Build history of the part. All positions in model axes, mm. A direction names the side the tool comes from. Round coordinates to 2 decimals unless told otherwise and drop trailing zeros. Write each loop counter-clockwise with the first axis right and the second up, starting at its lowest first coordinate (ties: lowest second). Pieces come first, ordered by that corner, then holes. Notation, with made-up numbers: (85, 84.5) - (116, 84.5) arc R10 cw to (116, 88.5) - close; hole circle Ø1 at (54, 15.5). An arc over 180 degrees is marked (long way). Answer as a JSON object with one key per item and string values. Group by question number.
Item 1: Slice it at A-A, the plane z = 0. List the corners of the cut face in (x, y) (3 decimals).
Item 2: Slice it at C-C, the plane x = 1.3. List the corners of the cut face in (y, z), then the cut area to 3 significant figures.
Item 3: Slice it at D-D, the plane y = -1.5. List the corners of the cut face in (x, z) (3 decimals), then the cut area to 3 significant figures.
Item 4: Which spindle directions (+Z, -Z, +X, -X, +Y, -Y) get a long thin tool onto all of the face, cutting with end or side? Do faces 4 (the flat face through (0, -2.8, 0)), 5 (the cylindrical face through (-0.75, 5.31, -0.03)), 6 (the cylindrical face through (1.092, -1.38, 0.344)), 7 (the flat face through (0, 7.2, 0)), 8 (the cylindrical face through (-1.4, 3.7, -0.06)). Say none if no direction does.
Item 5: Slice it at B-B, the plane z = 0.95. List the corners of the cut face in (x, y), then the cut area to 3 significant figures.
Item 6: Probe line 1 (Y direction, x = 0.9, z = 0.05); line 2 (Y direction, x = -1.2, z = -0.65); line 3 (Y direction, x = 1.8, z = 0.3). List the from-to ranges inside material, lowest first. Write a range as from..to.
Item 7: Flat gauge pins, fed straight in: pin 1 (1 mm diameter, centred on y = 0, z = 1, fed in from +X); pin 2 (1 mm diameter, centred on x = -1, z = -1.5, fed in from -Y); pin 3 (1.5 mm diameter, centred on y = 3.5, z = -0.5, fed in from -X). Where does each tip first touch, or does it go through?
Item 8: Two-plate mould, pull along Y, no slides. Class faces 1 (the cylindrical face through (-0.434, 0.345, 1.952)), 2 (the flat face through (0, 3.95, 1)), 3 (the flat face through (1, 0, 1)): +Y half, -Y half, draft (parallel to the pull), parting line (faces both ways), or undercut.
from build123d import *

# Parameters (mm, degrees)
SKETCH1_R           = 2
BOSS_EXTRUDE1_DEPTH = 0.7
SKETCH2_R           = 0.75
BOSS_EXTRUDE2_DEPTH = 2.75
SKETCH3_R           = 1.4
BOSS_EXTRUDE3_DEPTH = 0.5
SKETCH4_R           = 0.75
BOSS_EXTRUDE4_DEPTH = 2.75
SKETCH5_R           = 1.4
BOSS_EXTRUDE5_DEPTH = 0.5
SKETCH6_R           = 1.145
BOSS_EXTRUDE6_DEPTH = 2.8


with BuildPart() as part:
    # Sketch1 → Boss-Extrude1 (new body)
    with BuildSketch(Plane(origin=(0, 0, 0), x_dir=(1, 0, 0), z_dir=(0, 1, 0))):
        Circle(SKETCH1_R)
    extrude(amount=BOSS_EXTRUDE1_DEPTH)

    # Sketch2 → Boss-Extrude2 (add)
    with BuildSketch(Plane(origin=(0, 0.7, 0), x_dir=(1, 0, 0), z_dir=(0, 1, 0))):
        Circle(SKETCH2_R)
    extrude(amount=BOSS_EXTRUDE2_DEPTH)

    # Sketch3 → Boss-Extrude3 (add)
    with BuildSketch(Plane(origin=(0, 3.45, 0), x_dir=(1, 0, 0), z_dir=(0, 1, 0))):
        Circle(SKETCH3_R)
    extrude(amount=BOSS_EXTRUDE3_DEPTH)

    # Sketch4 → Boss-Extrude4 (add)
    with BuildSketch(Plane(origin=(0, 3.95, 0), x_dir=(1, 0, 0), z_dir=(0, 1, 0))):
        Circle(SKETCH4_R)
    extrude(amount=BOSS_EXTRUDE4_DEPTH)

    # Sketch5 → Boss-Extrude5 (add)
    with BuildSketch(Plane(origin=(0, 6.7, 0), x_dir=(1, 0, 0), z_dir=(0, 1, 0))):
        Circle(SKETCH5_R)
    extrude(amount=BOSS_EXTRUDE5_DEPTH)

    # Sketch6 → Boss-Extrude6 (add)
    with BuildSketch(Plane.XZ):
        Circle(SKETCH6_R)
    extrude(amount=BOSS_EXTRUDE6_DEPTH)


solid = part.part
Geometry says:
{
 "1": {"outline": "(-2, 0) - (-1.145, 0) - (-1.145, -2.8) - (1.145, -2.8) - (1.145, 0) - (2, 0) - (2, 0.7) - (0.75, 0.7) - (0.75, 3.45) - (1.4, 3.45) - (1.4, 3.95) - (0.75, 3.95) - (0.75, 6.7) - (1.4, 6.7) - (1.4, 7.2) - (-1.4, 7.2) - (-1.4, 6.7) - (-0.75, 6.7) - (-0.75, 3.95) - (-1.4, 3.95) - (-1.4, 3.45) - (-0.75, 3.45) - (-0.75, 0.7) - (-2, 0.7) - close"},
 "2": {"outline": "(0, -1.52) - (0.7, -1.52) - (0.7, 1.52) - (0, 1.52) - close; (3.45, -0.52) - (3.95, -0.52) - (3.95, 0.52) - (3.45, 0.52) - close; (6.7, -0.52) - (7.2, -0.52) - (7.2, 0.52) - (6.7, 0.52) - close", "area": "3.17 mm^2"},
 "3": {"outline": "circle Ø2.29 at (0, 0)", "area": "4.12 mm^2"},
 "4": {"face 4": "+Z, -Z, +X, -X, -Y", "face 5": "none", "face 6": "-Y", "face 7": "+Z, -Z, +X, -X, +Y", "face 8": "+Y"},
 "5": {"outline": "(-1.76, 0) - (-0.64, 0) - (-0.64, -2.8) - (0.64, -2.8) - (0.64, 0) - (1.76, 0) - (1.76, 0.7) - (-1.76, 0.7) - close; (-1.03, 3.45) - (1.03, 3.45) - (1.03, 3.95) - (-1.03, 3.95) - close; (-1.03, 6.7) - (1.03, 6.7) - (1.03, 7.2) - (-1.03, 7.2) - close", "area": "8.10 mm^2"},
 "6": {"line 1": "y = -2.8..0.7, 3.45..3.95, 6.7..7.2", "line 2": "y = 0..0.7, 3.45..3.95, 6.7..7.2", "line 3": "y = 0..0.7"},
 "7": {"pin 1": "stops at x = 1.94", "pin 2": "stops at y = 0", "pin 3": "stops at x = -1.4"},
 "8": {"face 1": "draft", "face 2": "undercut", "face 3": "-Y half"}
}
